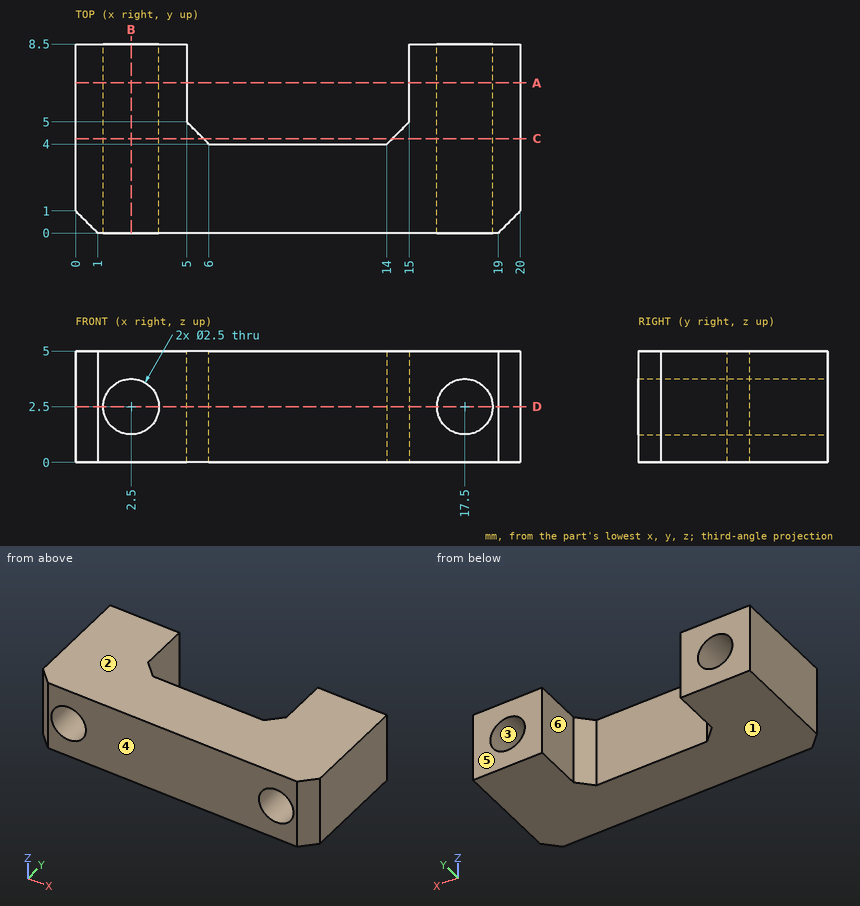
Could you check a few things on this drawing? It's one solid part, dimensions in mm from its lowest x, y, z. A direction names the side the tool comes from. Round coordinates to 2 decimals unless told otherwise and drop trailing zeros. Order: outer loops, then holes, each group sorted by start corner. A loop starts at its lowest first (then second) coordinate and runs counter-clockwise, first axis right, second up. Notation, with made-up numbers: M -17,6 L -13,6 A28 cw -13,41 Z; hole C 82,-29 d3. An arc over 180 degrees is marked long. Return JSON: item names as keys, results as strings. Group by question number.
1. On a 3-axis mill with a long thin cutter (end or side, diameter ignored), from which of +Z, -Z, +X, -X, +Y, -Y can I reach the whole of each face in a straight line? I mean the marked faces 5 and 6. Say none if no direction works.
2. Please list where these lines run through material, in increasing order: probe 1 along Z at (x, y) = (17.5, 5.5); probe 2 along X at (y, z) = (8, 4.6); probe 3 along Y at (x, z) = (8.75, 1.7).
3. If we section it at C-C on y = 4.25: List the corners of the cut face in (x, z) for me.
4. If we section it at A-A on y = 6.75: List the corners of the cut face in (x, z) for me.
5. If we mould it in two halves opening along Z, with no side actions, what happens to the marked faces 1, 2, 3 and 4? For each: pulls with the +Z half, pulls with the -Z half, needs draft (parallel to the pull), parting line crosses it, or undercut.
6. If we section it at B-B on x = 2.5: List the corners of the cut face in (y, z) for me, then the cut area to 4 significant figures.
7. If we section it at D-D on z = 2.5: List the corners of the cut face in (x, y) for me.
8. I'm going to push flat-ended pins straight in: pin 1 Ø2 at (x, z) = (2.5, 2.5) entering from -Y; pin 2 Ø1.5 at (x, z) = (11, 4) entering from +Y. Where does each tip first touch, or does it pass through?
Reply:
{
 "1": {"face 5": "+Z, -Z, +X, -X, +Y", "face 6": "+Z, -Z, +Y"},
 "2": {"probe 1": "0 to 1.25, 3.75 to 5", "probe 2": "0 to 5, 15 to 20", "probe 3": "0 to 4"},
 "3": {"outline": "M 0,0 L 5.75,0 L 5.75,5 L 0,5 Z; M 14.25,0 L 20,0 L 20,5 L 14.25,5 Z; hole C 2.5,2.5 d2.5; hole C 17.5,2.5 d2.5"},
 "4": {"outline": "M 0,0 L 5,0 L 5,5 L 0,5 Z; M 15,0 L 20,0 L 20,5 L 15,5 Z; hole C 2.5,2.5 d2.5; hole C 17.5,2.5 d2.5"},
 "5": {"face 1": "pulls with the -Z half", "face 2": "pulls with the +Z half", "face 3": "undercut", "face 4": "needs draft"},
 "6": {"outline": "M 0,0 L 8.5,0 L 8.5,1.25 L 0,1.25 Z; M 0,3.75 L 8.5,3.75 L 8.5,5 L 0,5 Z", "area": "21.25 mm^2"},
 "7": {"outline": "M 0,1 L 1,0 L 1.25,0 L 1.25,8.5 L 0,8.5 Z; M 3.75,0 L 16.25,0 L 16.25,8.5 L 15,8.5 L 15,5 L 14,4 L 6,4 L 5,5 L 5,8.5 L 3.75,8.5 Z; M 18.75,0 L 19,0 L 20,1 L 20,8.5 L 18.75,8.5 Z"},
 "8": {"pin 1": "through", "pin 2": "y = 4"}
}
